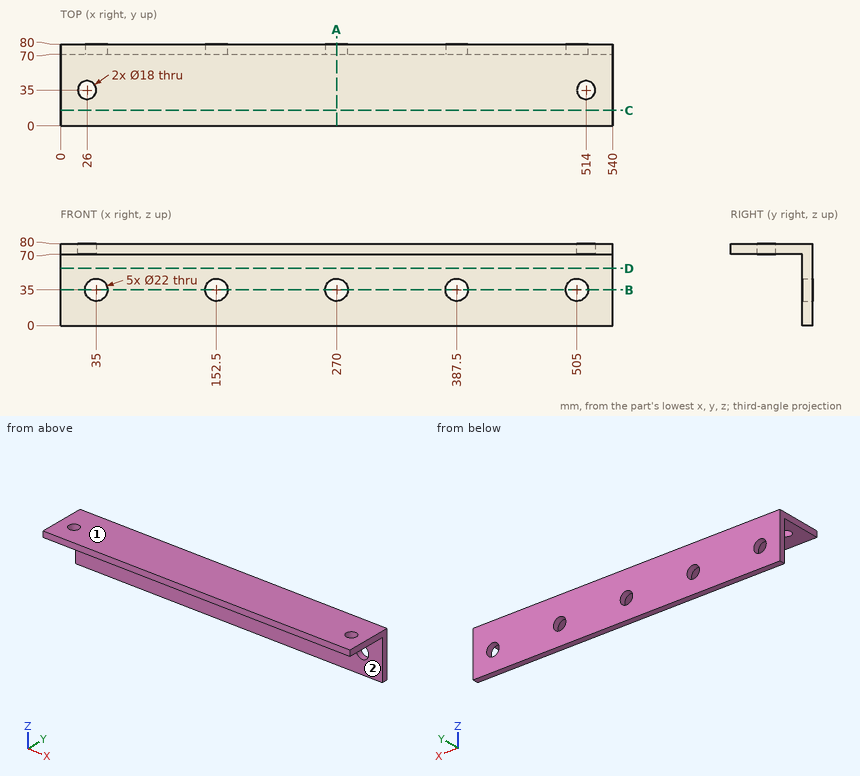
Print and shaded views of the part. All mm, measured from the part's lowest x, y and z. A direction names the side the tool comes from. Give positions to 0.01 mm unless a question says otherwise; leave off trailing zeros. Write each loop counter-clockwise with the first axis right and the second up, starting at its lowest first coordinate (ties: lowest second). Pieces come first, ordered by that corner, then holes. Notation, with made-up numbers: (-14, 86.5) -> (5, 86.5) arc R7 ccw to (5, 95.5) -> close; hole circle Ø4 at (2, 85). An arc over 180 degrees is marked (long way). Write item = value, one per line.
(1) Slice it at C-C, the plane y = 15. Give the cut face in (x, z).
Determined:
outline = (0, 70) -> (540, 70) -> (540, 80) -> (0, 80) -> close
(2) Slice it at B-B, the plane z = 35. Give the cut face in (x, y), then the cut area to 3 significant figures.
Determined:
outline = (0, 70) -> (24, 70) -> (24, 80) -> (0, 80) -> close; (46, 70) -> (141.5, 70) -> (141.5, 80) -> (46, 80) -> close; (163.5, 70) -> (259, 70) -> (259, 80) -> (163.5, 80) -> close; (281, 70) -> (376.5, 70) -> (376.5, 80) -> (281, 80) -> close; (398.5, 70) -> (494, 70) -> (494, 80) -> (398.5, 80) -> close; (516, 70) -> (540, 70) -> (540, 80) -> (516, 80) -> close
area = 4,300 mm2
(3) Tool access for the marked faces 1 and 2: list every direction of +Z, -Z, +X, -X, +Y, -Y with a clear straight run to the whole face (end or side of a thin tool).
Determined:
face_1 = +Z, +X, -X, +Y, -Y
face_2 = -Z, +X, -X, -Y
(4) Flat gauge pins, fed straight in: P1, Ø23.5, axis at x = 26, y = 35, coming from the -Z side; P2, Ø8, axis at x = 69.5, z = 25, coming from the -Y side; P3, Ø20, axis at x = 35, z = 35, coming from the -Y side. Where does each tip first touch, or does it go through?
Determined:
P1 = 70
P2 = 70
P3 = through
(5) Probe line 1 along Z through (x, y) = (388, 74); line 2 along Y through (x, z) = (26, 76.25); line 3 along X through (y, z) = (37, 74). List the from-to ranges inside material, lowest first.
Determined:
line_1 = 0 to 24.01, 45.99 to 80
line_2 = 0 to 26, 44 to 80
line_3 = 0 to 17.23, 34.77 to 505.23, 522.77 to 540
(6) Slice it at A-A, the plane x = 270. Give the cut face in (y, z), then the cut area to 3 significant figures.
Determined:
outline = (0, 70) -> (70, 70) -> (70, 46) -> (80, 46) -> (80, 80) -> (0, 80) -> close; (70, 0) -> (80, 0) -> (80, 24) -> (70, 24) -> close
area = 1,280 mm2
